```python
from build123d import *

# Parameters (mm, degrees)
SWEEP1_PROFILE_R = 25.4
SHELL1_T         = -2.54


with BuildPart() as part:
    # Sweep1: sweep along a curve in space
    with BuildLine() as sweep1_path:
        Line((0, 254, 0), (177.8, 254, 0))
        ThreePointArc((177.8, 254, 0), (231.681536726, 254, 22.318463274), (254, 254, 76.2))
        Line((254, 254, 76.2), (254, 254, 177.8))
        ThreePointArc((254, 254, 177.8), (254, 231.681536726, 231.681536726), (254, 177.8, 254))
        Line((254, 177.8, 254), (254, 0, 254))
    # Sweep1 profile (on start of the path) → Sweep1 (sweep)
    with BuildSketch(Plane(origin=(0, 254, 0), x_dir=(0, 0, 1), z_dir=(1, 0, 0))):
        Circle(SWEEP1_PROFILE_R)
    sweep(path=sweep1_path.line)

    # Shell1
    shell1_openings = [part.faces().sort_by_distance(p)[0] for p in [
        (254, 0, 254),
        (0, 254, 0),
    ]]
    offset(amount=SHELL1_T, openings=shell1_openings, kind=Kind.INTERSECTION)


solid = part.part
```
The listing builds one solid part. Answer for the finished solid, in the listing's coordinates (mm). A direction names the side the tool comes from. Give positions to 0.01 mm unless a question says otherwise; leave off trailing zeros. Order: outer loops, then holes, each group sorted by start corner. A loop starts at its lowest first (then second) coordinate and runs counter-clockwise, first axis right, second up.
Item 1: Find the intervals of material crossed by probe 1 along Z at (x, y) = (59, 254); probe 2 along Y at (x, z) = (254, 147); probe 3 along Z at (x, y) = (62, 252), in increasing order.
From the geometry:
probe 1: z = -25.4 to -22.86, 22.86 to 25.4
probe 2: y = 228.6 to 231.14, 276.86 to 279.4
probe 3: z = -25.32 to -22.77, 22.77 to 25.32
Item 2: The part is cut by section A-A, the plane y = 170.5. Give the vertices of the cut face in (x, z), and give its area (3 significant figures).
From the geometry:
outline: circle Ø50.8 at (254, 254); hole circle Ø45.72 at (254, 254)
area: 385 mm2
Item 3: The part is cut by section B-B, the plane x = 161. Give the vertices of the cut face in (y, z), and give its area (3 significant figures).
From the geometry:
outline: circle Ø50.8 at (254, 0); hole circle Ø45.72 at (254, 0)
area: 385 mm2
Item 4: For a pull along Y with two mould halves and no side action, classify faces 1 (the face through (256.976, 231.335, 127.711)), 2 (the face through (256.976, 87.655, 231.335)), 3 (the face through (90.145, 278.796, -5.506)), 4 (the face through (264, 0, 275)) as pulls with the +Y half, pulls with the -Y half, needs draft (parallel to the pull), parting line crosses it, or undercut.
From the geometry:
face 1: undercut
face 2: needs draft
face 3: parting line crosses it
face 4: pulls with the -Y half
Item 5: Given pin 1 Ø12 at (y, z) = (247.5, 178) entering from +X; pin 2 Ø12 at (x, z) = (240, 82.5) entering from +Y, each flat-ended and moving along its own axis, determine where each tip first touches the part or whether it passes through.
From the geometry:
pin 1: stops at x = 279.4
pin 2: stops at y = 278.11
Item 6: Which of the six approach directions +Z, -Z, +X, -X, +Y, -Y give full straight-line access (tool end or side, diameter ignored) to faces 5 (the face through (0, 244, -21)), 6 (the face through (259.506, 278.796, 127.711)), 7 (the face through (259.506, 87.655, 278.796)), 8 (the face through (90.145, 231.335, -2.976))?
From the geometry:
face 5: +Z, -Z, -X, +Y, -Y
face 6: none
face 7: -Y
face 8: -X
